Design review of the part shown in the three views and the two pictorial views. Dimensions are in mm from the part's minimum x, y and z. A direction names the side the tool comes from. Coordinates: 2 decimals unless noted, no trailing zeros. Write each loop counter-clockwise with the first axis right and the second up, starting at its lowest first coordinate (ties: lowest second). Pieces come first, ordered by that corner, then holes. Notation, with made-up numbers: (55, 4.25) - (104, 4.25) arc R12 cw to (104, 12.25) - close; hole circle Ø1 at (50.25, 15). An arc over 180 degrees is marked (long way). Return JSON: item names as keys, results as strings. Group by question number.
(1) Tool access review of the marked faces 1, 2 and 3: name each direction out of +Z, -Z, +X, -X, +Y, -Y from which nothing blocks a thin tool from reaching the whole face with its end or side.
(2) For pin 1 Ø10 at (x, y) = (41.5, 33.5) entering from +Z; pin 2 Ø4 at (x, z) = (44, 12.5) entering from -Y; pin 3 Ø24 at (x, y) = (14.5, 14.5) entering from +Z; pin 4 Ø3 at (x, z) = (18, 30) entering from -Y, all flat-tipped, find the tip position at first contact; note any pin that passes through.
(3) To check wall thickness, follow L1, parallel to Z at x = 44, y = 3; L2, parallel to Y at x = 19, z = 28; L3, parallel to X at y = 33.5, z = 16. State the ranges of each line that lie inside material, in increasing order. Write a range as from..to.
(4) We need section D-D on y = 9.5. State the section outline as (x, z) points.
(5) We need section B-B on x = 17.5. State the section outline as (y, z) points.
(6) We need section A-A on y = 31.5. State the section outline as (x, z) points.
(7) We need section C-C on z = 33.5. State the section outline as (x, y) points.
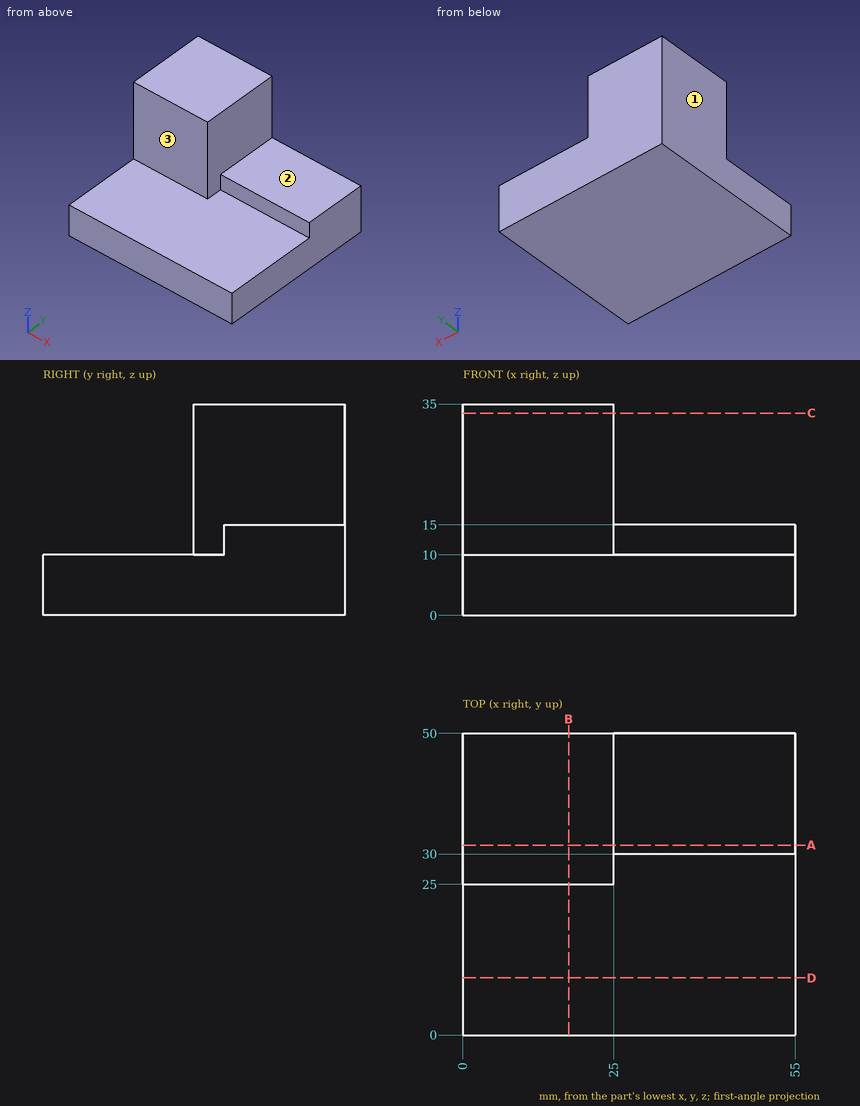
Ans:
{
 "1": {"face 1": "+Z, -Z, -X, +Y, -Y", "face 2": "+Z, +X, +Y, -Y", "face 3": "+Z, +X, -X, -Y"},
 "2": {"pin 1": "z = 15", "pin 2": "y = 30", "pin 3": "z = 35", "pin 4": "y = 25"},
 "3": {"L1": "0..10", "L2": "25..50", "L3": "0..25"},
 "4": {"outline": "(0, 0) - (55, 0) - (55, 10) - (0, 10) - close"},
 "5": {"outline": "(0, 0) - (50, 0) - (50, 35) - (25, 35) - (25, 10) - (0, 10) - close"},
 "6": {"outline": "(0, 0) - (55, 0) - (55, 15) - (25, 15) - (25, 35) - (0, 35) - close"},
 "7": {"outline": "(0, 25) - (25, 25) - (25, 50) - (0, 50) - close"}
}
